```python
from build123d import *

# Parameters (mm, degrees)
SKETCH1_W                                      = 40
SKETCH1_H                                      = 49
SKETCH1_W_2                                    = 30
SKETCH1_H_2                                    = 30
BOSS_EXTRUDE1_DEPTH                            = 3
FILLET1_R                                      = 5
CSK_FOR_M4_FLAT_HEAD_MACHINE_SCREW2_AT_2_COUNT = 2
CSK_FOR_M4_FLAT_HEAD_MACHINE_SCREW2_AT_2_PITCH = 30
CSK_FOR_M4_FLAT_HEAD_MACHINE_SCREW2_AT_3_COUNT = 2
CSK_FOR_M4_FLAT_HEAD_MACHINE_SCREW2_AT_3_PITCH = 42.426406871
CSK_FOR_M4_FLAT_HEAD_MACHINE_SCREW2_AT_4_COUNT = 2
CSK_FOR_M4_FLAT_HEAD_MACHINE_SCREW2_AT_4_PITCH = 30
SKETCH4_R                                      = 6
CUT_EXTRUDE1_DEPTH                             = 3


with BuildPart() as part:
    # Sketch1 → Boss-Extrude1 (new body)
    # profile 1 of 2: a face of its own
    with BuildSketch(Plane(origin=(0, 0, 0), x_dir=(1, 0, 0), z_dir=(0, 1, 0))):
        with Locations((20, 24.5)):
            Rectangle(SKETCH1_W, SKETCH1_H)
        with Locations((20, 29)):
            Rectangle(SKETCH1_W_2, SKETCH1_H_2, mode=Mode.SUBTRACT)
    # profile 2 of 2: a face of its own
    with BuildSketch(Plane(origin=(0, 0, 0), x_dir=(1, 0, 0), z_dir=(0, 1, 0))):
        with Locations((20, 29)):
            Rectangle(SKETCH1_W_2, SKETCH1_H_2)
    extrude(amount=BOSS_EXTRUDE1_DEPTH)

    # Fillet1
    # the kernel refuses this fillet: 5 mm, written as the material it takes off along each edge
    with BuildSketch(Plane(origin=(-11.456439237, 3, 0), x_dir=(0, -1, 0), z_dir=(1, 0, 0))) as fillet1_piece_1:
        with BuildLine():
            CenterArc((5, 4.582575695), FILLET1_R, 180, 66.421821522)
            Line((0, 4.582575695), (-0.1, 4.582575695))
            Line((-0.1, 4.582575695), (-0.1, 0))
            Line((-0.1, 0), (0, -0.1))
            ThreePointArc((0, -0.1), (1.5, -0.1), (2.96, -0.091651514))
            Line((2.96, -0.091651514), (3, 0))
        make_face()
    extrude(amount=62.912878475, mode=Mode.SUBTRACT)
    with BuildSketch(Plane(origin=(0, -12.5, -49), x_dir=(0, 0, 1), z_dir=(0, 1, 0))) as fillet1_piece_2:
        with BuildLine():
            CenterArc((FILLET1_R, FILLET1_R), FILLET1_R, 180, 90)
            Line((0, FILLET1_R), (-FILLET1_R * 0.02, FILLET1_R))
            Line((-FILLET1_R * 0.02, FILLET1_R), (-FILLET1_R * 0.02, -FILLET1_R * 0.02))
            Line((-FILLET1_R * 0.02, -FILLET1_R * 0.02), (FILLET1_R, -FILLET1_R * 0.02))
            Line((FILLET1_R, -FILLET1_R * 0.02), (FILLET1_R, 0))
        make_face()
    extrude(amount=28, mode=Mode.SUBTRACT)
    with BuildSketch(Plane(origin=(40, -12.5, -49), x_dir=(0, 0, 1), z_dir=(0, 1, 0))) as fillet1_piece_3:
        with BuildLine():
            CenterArc((FILLET1_R, -FILLET1_R), FILLET1_R, 90, 90)
            Line((0, -FILLET1_R), (-FILLET1_R * 0.02, -FILLET1_R))
            Line((-FILLET1_R * 0.02, -FILLET1_R), (-FILLET1_R * 0.02, FILLET1_R * 0.02))
            Line((-FILLET1_R * 0.02, FILLET1_R * 0.02), (FILLET1_R, FILLET1_R * 0.02))
            Line((FILLET1_R, FILLET1_R * 0.02), (FILLET1_R, 0))
        make_face()
    extrude(amount=28, mode=Mode.SUBTRACT)

    # Sketch3 → CSK for M4 Flat Head Machine Screw2 (revolve, cut)
    with BuildSketch(Plane(origin=(5, 3, -44), x_dir=(0, 0, 1), z_dir=(1, 0, 0))):
        Polygon((0, 0), (0, 3), (2.25, 3), (2.25, 2.45), (4.7, 0), align=None)
    csk_for_m4_flat_head_machine_screw2 = revolve(axis=Axis((5, 9.35, -44), (0, -1, 0)), mode=Mode.SUBTRACT)

    # CSK for M4 Flat Head Machine Screw2 at 2: CSK for M4 Flat Head Machine Screw2 ×2
    with Locations(*[(i * CSK_FOR_M4_FLAT_HEAD_MACHINE_SCREW2_AT_2_PITCH, 0, 0) for i in range(1, CSK_FOR_M4_FLAT_HEAD_MACHINE_SCREW2_AT_2_COUNT)]):
        add(csk_for_m4_flat_head_machine_screw2, mode=Mode.SUBTRACT)

    # CSK for M4 Flat Head Machine Screw2 at 3: CSK for M4 Flat Head Machine Screw2 ×2
    with Locations(*[Vector(0.7071067811865474, 0, 0.7071067811865477) * (i * CSK_FOR_M4_FLAT_HEAD_MACHINE_SCREW2_AT_3_PITCH) for i in range(1, CSK_FOR_M4_FLAT_HEAD_MACHINE_SCREW2_AT_3_COUNT)]):
        add(csk_for_m4_flat_head_machine_screw2, mode=Mode.SUBTRACT)

    # CSK for M4 Flat Head Machine Screw2 at 4: CSK for M4 Flat Head Machine Screw2 ×2
    with Locations(*[(0, 0, i * CSK_FOR_M4_FLAT_HEAD_MACHINE_SCREW2_AT_4_PITCH) for i in range(1, CSK_FOR_M4_FLAT_HEAD_MACHINE_SCREW2_AT_4_COUNT)]):
        add(csk_for_m4_flat_head_machine_screw2, mode=Mode.SUBTRACT)

    # Sketch4 → Cut-Extrude1 (cut)
    with BuildSketch(Plane(origin=(0, 3, 0), x_dir=(1, 0, 0), z_dir=(0, 1, 0))):
        with Locations(Location((20, 29, 0), (0, 0, 270))):
            Circle(SKETCH4_R)
    extrude(amount=-CUT_EXTRUDE1_DEPTH, mode=Mode.SUBTRACT)


solid = part.part
```
Check sheet for the modelled part. Datum: model origin and axes. Units: mm. Give positions to 0.01 mm unless a question says otherwise; leave off trailing zeros. Loops run counter-clockwise (first coordinate to the right, second up) from the corner with the lowest first, then second, coordinate; pieces in that order, holes last. Notation, with made-up numbers: M 4.5,77.25 L 32.5,77.25 A21 ccw 32.5,94.25 Z; hole C 28.25,-35.5 d5. An arc over 180 degrees is marked long. Answer in a Markdown table with one row per item.
1) Mould release check, pull along X, two halves, no side actions. Record for faces 1 (the face through (0, 1, -22)), 2 (the face through (32.77, 0.28, -14.29)), 3 (the face through (19.72, 2.205, -1.878)), 4 (the face through (39, 1, -47)): released by +X, released by -X, zero draft, split by the parting line, or undercut.
Solutions:
| item | result |
|---|---|
| face 1 | released by -X |
| face 2 | undercut |
| face 3 | zero draft |
| face 4 | released by +X |
2) Thickness scan on line 1 (X direction, y = 0.35, z = -44); line 2 (Z direction, x = 35, y = 0.75); line 3 (Z direction, x = 2, y = 1.85). Record the ranges inside material, lowest first.
Solutions:
| item | result |
|---|---|
| line 1 | x = 0 to 2.75, 7.25 to 32.75, 37.25 to 40 |
| line 2 | z = -49 to -46.45, -41.55 to -16.45, -11.55 to -0.41 |
| line 3 | z = -48 to -45.9, -42.1 to -15.9, -12.1 to -1.39 |
3) Cross-section at A-A (z = -29). Enter the section's corners in (x, y), plus the area to 3 significant figures.
Solutions:
| item | result |
|---|---|
| outline | M 0,0 L 14,0 L 14,3 L 0,3 Z; M 26,0 L 40,0 L 40,3 L 26,3 Z |
| area | 84.0 mm^2 |
4) Cross-section at B-B (x = 16). Enter the section's corners in (y, z).
Solutions:
| item | result |
|---|---|
| outline | M 0,-49 L 3,-49 L 3,-33.47 L 0,-33.47 Z; M 0,-24.53 L 3,-24.53 L 3,-4.58 A5 ccw 0,0 Z |
5) Cross-section at C-C (z = -14). Enter the section's corners in (x, y), plus the area to 3 significant figures.
Solutions:
| item | result |
|---|---|
| outline | M 0,0 L 2.75,0 L 2.75,0.55 L 0.3,3 L 0,3 Z; M 7.25,0 L 32.75,0 L 32.75,0.55 L 30.3,3 L 9.7,3 L 7.25,0.55 Z; M 37.25,0 L 40,0 L 40,3 L 39.7,3 L 37.25,0.55 Z |
| area | 81.0 mm^2 |
6) Cross-section at D-D (y = 1.4). Enter the section's corners in (x, z).
Solutions:
| item | result |
|---|---|
| outline | M 0,-44 A5 ccw 5,-49 L 35,-49 A5 ccw 40,-44 L 40,-0.92 L 0,-0.92 Z; hole C 5,-44 d6.2; hole C 5,-14 d6.2; hole C 20,-29 d12; hole C 35,-44 d6.2; hole C 35,-14 d6.2 |
